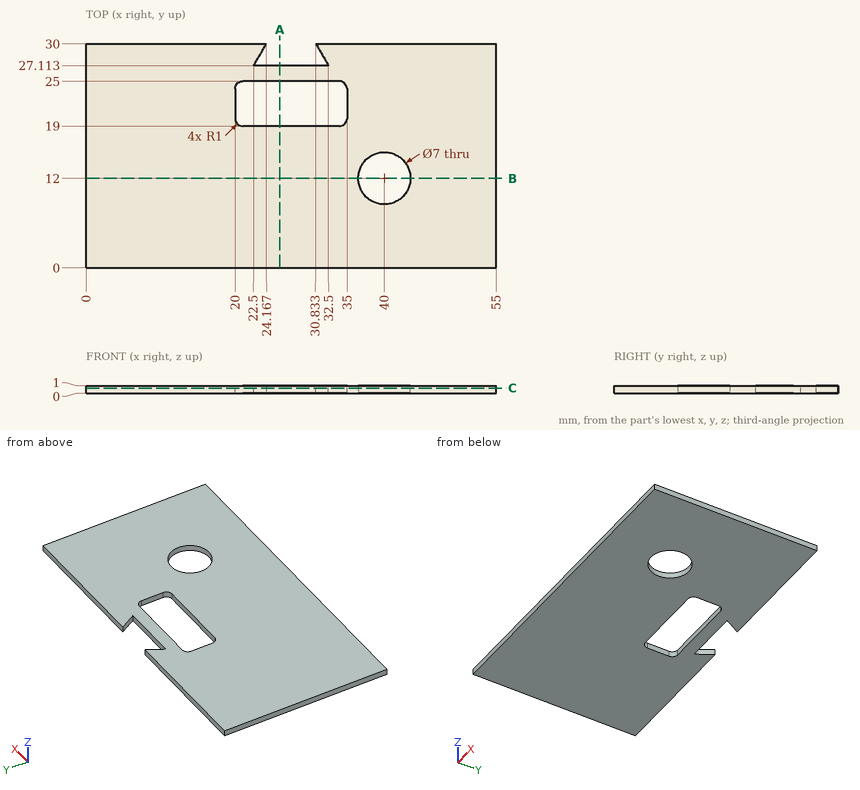
Could you check a few things on this drawing? It's one solid part, dimensions in mm from its lowest x, y, z. Round coordinates to 2 decimals unless told otherwise and drop trailing zeros. Loops run counter-clockwise (first coordinate to the right, second up) from the corner with the lowest first, then second, coordinate; pieces in that order, holes last.
Q1. Please list where these lines run through material, in increasing order: L1, parallel to X at y = 12, z = 0.7; L2, parallel to Y at x = 25, z = 0.4; L3, parallel to X at y = 21, z = 0.7.
Q2. I want a section at C-C (z = 0.7). Write out the boundary of the cut face in (x, y).
Q3. I want a section at A-A (x = 26). Write out the boundary of the cut face in (y, z), and give its area (3 significant figures).
Q4. I want a section at B-B (y = 12). Write out the boundary of the cut face in (x, z).
Answer below:
1. L1: x = 0 to 36.5, 43.5 to 55
1. L2: y = 0 to 19, 25 to 27.11
1. L3: x = 0 to 20, 35 to 55
2. outline: (0, 0) - (55, 0) - (55, 30) - (30.83, 30) - (32.5, 27.11) - (22.5, 27.11) - (24.17, 30) - (0, 30) - close; hole (20, 20) arc R1 ccw to (21, 19) - (34, 19) arc R1 ccw to (35, 20) - (35, 24) arc R1 ccw to (34, 25) - (21, 25) arc R1 ccw to (20, 24) - close; hole circle Ø7 at (40, 12)
3. outline: (0, 0) - (19, 0) - (19, 1) - (0, 1) - close; (25, 0) - (27.11, 0) - (27.11, 1) - (25, 1) - close
3. area: 21.1 mm2
4. outline: (0, 0) - (36.5, 0) - (36.5, 1) - (0, 1) - close; (43.5, 0) - (55, 0) - (55, 1) - (43.5, 1) - close
